```python
from build123d import *

# Parameters (mm, degrees)
F0_R     = 2.5
F0_R_2   = 1.5
F1_DEPTH = 5
F0_R_3   = 4
F0_R_4   = 3
F2_DEPTH = 1
F3_DEPTH = 7
F4_R     = 2
F5_DEPTH = 25


with BuildPart() as f1:
    # F0 (on Front) → F1 (new body)
    with BuildSketch(Plane.XZ):
        Circle(F0_R)
        Circle(F0_R_2, mode=Mode.SUBTRACT)
    extrude(amount=-F1_DEPTH)

    # F0 (on Front) → F2 (join)
    with BuildSketch(Plane.XZ):
        Circle(F0_R_3)
        Circle(F0_R_4, mode=Mode.SUBTRACT)
        Circle(F0_R_4)
        Circle(F0_R, mode=Mode.SUBTRACT)
        Circle(F0_R)
        Circle(F0_R_2, mode=Mode.SUBTRACT)
    extrude(amount=F2_DEPTH)

    # F0 (on Front) → F3 (join)
    with BuildSketch(Plane.XZ):
        Circle(F0_R_3)
        Circle(F0_R_4, mode=Mode.SUBTRACT)
    extrude(amount=F3_DEPTH)

    # F4 (on Top) → F5 (cut)
    with BuildSketch(Plane.XY):
        with Locations((0, -3.5)):
            Circle(F4_R)
    extrude(amount=F5_DEPTH, mode=Mode.SUBTRACT)


solid = f1.part
```
CAD build for the part. Positions are in the model's coordinates, mm. A direction names the side the tool comes from. Give positions to 0.01 mm unless a question says otherwise; leave off trailing zeros. Order: outer loops, then holes, each group sorted by start corner. A loop starts at its lowest first (then second) coordinate and runs counter-clockwise, first axis right, second up. Notation, with made-up numbers: M 38,-2.75 L 81,-2.75 A24 cw 81,22.25 Z; hole C 66,0.5 d2. An arc over 180 degrees is marked long. Put each result on its own line as item: value. Start each with the question number.
(1) Saw through at B-B, the plane z = 0. Write the cut outline in (x, y), then the cut area to 3 significant figures.
(2) Saw through at D-D, the plane y = -0.5. Write the cut outline in (x, z).
(3) Drill centre lines: line 1 along Z through (x, y) = (0, 2.45); line 2 along Y through (x, z) = (-1.5, -2.75); line 3 along Y through (x, z) = (0, 2.8). Where is each one in solid material? Low to high.
(4) Which spindle directions (+Z, -Z, +X, -X, +Y, -Y) get a long thin tool onto all of the face, cutting with end or side? Do faces 1 (the cylindrical face through (-0.867, -3.451, -3.905)), 2 (the flat face through (2, 0, 2)), 3 (the cylindrical face through (-0.65, -3.96, -2.93)). Say none if no direction does.
(5) Saw through at A-A, the plane x = 0. Write the cut outline in (y, z), then the cut area to 3 significant figures.
(6) Saw through at C-C, the plane x = -2.75. Write the cut outline in (y, z), then the cut area to 3 significant figures.
(7) Mould opens along X. For faces 4 (the cylindrical face through (1.908, -2.899, 3.106)), 5 (the flat face through (1, -7, 3)), 6 (the cylindrical face through (-0.54, 2.46, -2.44)), 7 (the cylindrical face through (-1.5, 2.04, 0.07)) say: +X half, -X half, draft (parallel to the pull), parting line (faces both ways), or undercut.
(8) Flat gauge pins, fed straight in: pin 1 Ø1.8 at (x, z) = (0, 0) entering from -Y; pin 2 Ø1.5 at (x, z) = (1, -1.5) entering from -Y; pin 3 Ø2 at (y, z) = (-2.5, -2.5) entering from +X. Where does each tip first touch, or does it go through?
Check result:
1. outline: M -4,-7 L -3,-7 L -3,-1 L -1.5,-1 L -1.5,5 L -2.5,5 L -2.5,0 L -4,0 Z; M 1.5,-1 L 3,-1 L 3,-7 L 4,-7 L 4,0 L 2.5,0 L 2.5,5 L 1.5,5 Z
1. area: 27.0 mm2
2. outline: C 0,0 d8; hole C 0,0 d3
3. line 1: z = -2.5 to -1.5, 1.5 to 2.5
3. line 2: y = -7 to 0
3. line 3: y = -1 to 0
4. face 1: +Y, -Y
4. face 2: +Y
4. face 3: -Y
5. outline: M -7,-4 L 0,-4 L 0,-2.5 L 5,-2.5 L 5,-1.5 L -1,-1.5 L -1,-3 L -7,-3 Z; M -7,3 L -5.5,3 L -5.5,4 L -7,4 Z; M -1.5,3 L -1,3 L -1,1.5 L 5,1.5 L 5,2.5 L 0,2.5 L 0,4 L -1.5,4 Z
5. area: 23.0 mm2
6. outline: M -7,-2.9 L 0,-2.9 L 0,2.9 L -7,2.9 L -7,1.2 L -1,1.2 L -1,-1.2 L -7,-1.2 Z
6. area: 26.3 mm2
7. face 4: undercut
7. face 5: draft
7. face 6: parting line
7. face 7: undercut
8. pin 1: passes through
8. pin 2: stops at y = -1
8. pin 3: stops at x = 3.71
